Here's the drawing with two shaded views (mm, measured from the low corner). I have some questions. A direction names the side the tool comes from. Round coordinates to 2 decimals unless told otherwise and drop trailing zeros. Loops run counter-clockwise (first coordinate to the right, second up) from the corner with the lowest first, then second, coordinate; pieces in that order, holes last.
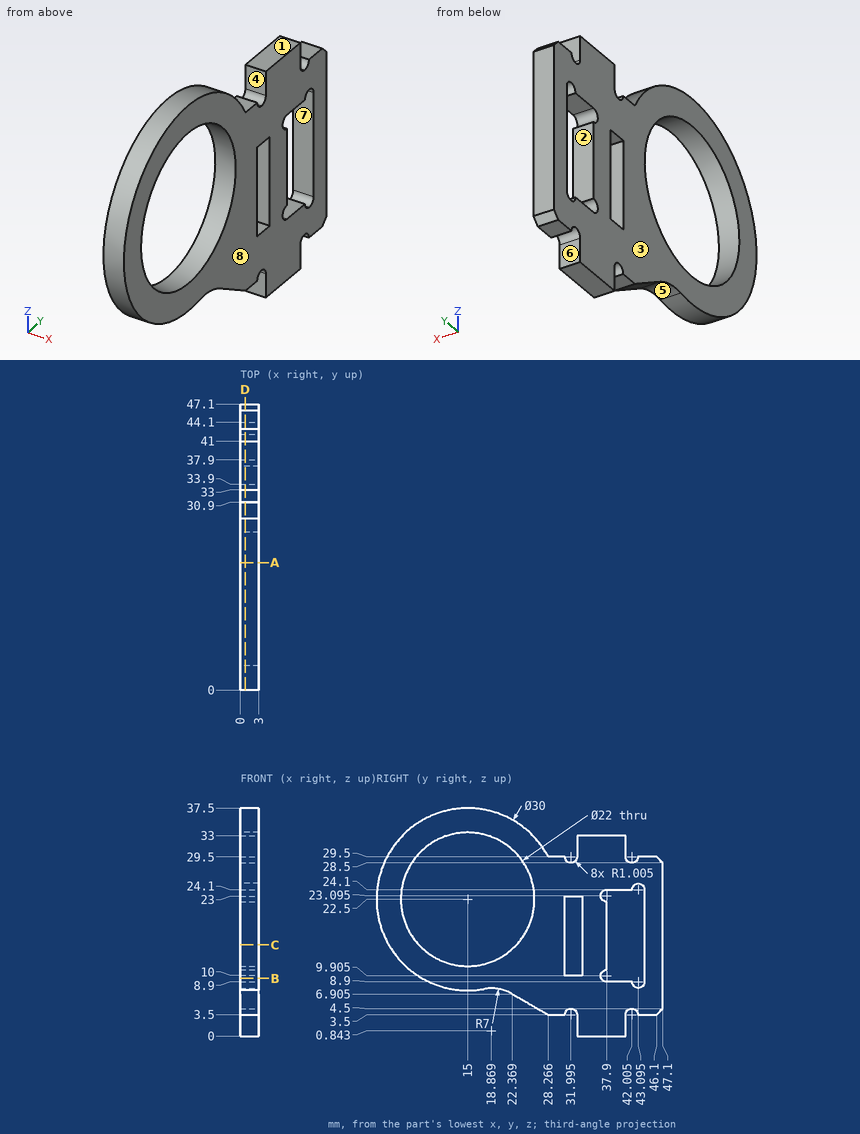
(1) If we section it at C-C, the plane z = 15: List the corners of the cut face in (x, y) for me.
Worked answers:
outline: (0, 2.01) - (3, 2.01) - (3, 6.95) - (0, 6.95) - close; (0, 23.05) - (3, 23.05) - (3, 30.9) - (0, 30.9) - close; (0, 33.9) - (3, 33.9) - (3, 37.9) - (0, 37.9) - close; (0, 44.1) - (3, 44.1) - (3, 47.1) - (0, 47.1) - close
(2) Will these pins go through, and if not, where does the flat tip stop? P1, Ø0.9, axis at x = 2, z = 17, coming from the -Y side (1 decimal); P2, Ø1, axis at y = 13.5, z = 14, coming from the -X side; P3, Ø1.5, axis at x = 1, z = 1.5, coming from the +Y side; P4, Ø0.8, axis at x = 1, y = 29, coming from the +Z side.
Worked answers:
P1: stops at y = 0.9
P2: passes through
P3: stops at y = 41
P4: stops at z = 29.5
(3) If we section it at B-B, the plane z = 9.5: List the corners of the cut face in (x, y) for me.
Worked answers:
outline: (0, 7.52) - (3, 7.52) - (3, 36.98) - (0, 36.98) - close; (0, 44.1) - (3, 44.1) - (3, 47.1) - (0, 47.1) - close
(4) If we mould it in two halves opening along Y, with no side actions, what happens to the marked faces 6, 7 and 8? For each: released by +Y, released by -Y, zero draft, split by the parting line, or undercut.
Worked answers:
face 6: released by +Y
face 7: undercut
face 8: zero draft
(5) If I drill on line 1 (Z direction, x = 0.45, y = 38); line 2 (Y direction, x = 0.8, z = 22.5); line 3 (Y direction, x = 1.3, z = 31) (1 decimal), over which ranges is the centre line in solid material (lowest first)?
Worked answers:
line 1: z = 0 to 8.9, 24.1 to 33
line 2: y = 0 to 4, 26 to 30.9, 33.9 to 37.09, 44.1 to 47.1
line 3: y = 2.6 to 8, 22 to 27.4, 33 to 41
(6) For the marked faces 1, 2, 3, 4 and 5, which set-ups out of +Z, -Z, +X, -X, +Y, -Y let a thin tool reach every point of the face, with its end or its side?
Worked answers:
face 1: +Z, +X, -X, +Y
face 2: +X, -X
face 3: +Z, -Z, -X, +Y, -Y
face 4: +Z, +X, -X
face 5: -Z, +X, -X
(7) If we section it at D-D, the plane x = 0.8: State how many separate pieces and enclosed holes the cut face has.
Worked answers:
separate pieces: 1
enclosed holes: 3
(8) If we section it at A-A, the plane y = 21: List the corners of the cut face in (x, z) for me, then the cut area to 3 significant figures.
Worked answers:
outline: (0, 7.51) - (3, 7.51) - (3, 13.28) - (0, 13.28) - close; (0, 31.72) - (3, 31.72) - (3, 36.25) - (0, 36.25) - close
area: 30.9 mm2
